Read the model definition and answer for the solid it produces. Units are mm, in the model's axes. Face numbers are marked on the shaded views. Coordinates: 2 decimals unless noted, no trailing zeros. Order: outer loops, then holes, each group sorted by start corner. A loop starts at its lowest first (then second) coordinate and runs counter-clockwise, first axis right, second up. Notation, with made-up numbers: (73, 71.5) -> (95, 71.5) arc R19 ccw to (95, 82.5) -> close; hole circle Ø9 at (-10.75, -17.75). An arc over 180 degrees is marked (long way). Answer as a JSON object with one key per item and string values. Group by question number.
1) Determine the mould class of the marked faces 1 and 2 for opening direction X: released by +X, released by -X, zero draft, split by the parting line, or undercut.
2) Section C-C on y = 119 is taken. Determine the outline of the cut face in (x, z), and give its area (3 significant figures).
3) Section A-A on x = 0 is taken. Determine the outline of the cut face in (y, z), and give its area (3 significant figures).
4) Given pin 1 (3 mm diameter, centred on y = 70.5, z = 4, fed in from -X); pin 2 (2 mm diameter, centred on x = 10, y = 101.5, fed in from +Z); pin 3 (1.5 mm diameter, centred on x = -7, y = 53, fed in from +Z), each flat-ended and moving along its own axis, determine where each tip first touches the part or whether it passes through.
5) Consider L1, parallel to X at y = 98, z = -0.25; L2, parallel to Z at x = 1.75, y = 81; L3, parallel to X at y = 50.5, z = 3.25. Determine where each line is inside the solid, lowest interval first.
6) Section B-B on z = 0 is taken. Determine the outline of the cut face in (x, y).
from build123d import *
from OCP.BRepFilletAPI import BRepFilletAPI_MakeChamfer

# Parameters (mm, degrees)
SKETCH1_R           = 15
BOSS_EXTRUDE1_DEPTH = 153.775561
SKETCH2_R           = 8.083843349
CUT_EXTRUDE1_DEPTH  = 156.231836815
CHAMFER1_SIZE       = 3.249874
CHAMFER1_SIZE2      = 2.3566


with BuildPart() as part:
    # Sketch1 → Boss-Extrude1 (new body)
    with BuildSketch(Plane(origin=(0, 0, 0), x_dir=(1, 0, 0), z_dir=(0, 1, 0))):
        with Locations(Location((0, 0, 0), (0, 0, 270))):
            Circle(SKETCH1_R)
    extrude(amount=BOSS_EXTRUDE1_DEPTH)

    # Sketch2 → Cut-Extrude1 (cut, through all)
    with BuildSketch(Plane(origin=(0, 0, 0), x_dir=(1, 0, 0), z_dir=(0, 1, 0))):
        with Locations(Location((0, 0, 0), (0, 0, 270))):
            Circle(SKETCH2_R)
    extrude(amount=CUT_EXTRUDE1_DEPTH, mode=Mode.SUBTRACT)

    # Chamfer1: one chamfer whose edges measure the first distance from different faces: ONE call of the kernel's chamfer builder (chamfer() names one face for all edges)
    chamfer1_edges_1 = [part.edges().sort_by_distance(p)[0] for p in [
        (0, 0, -15),
    ]]
    chamfer1_side_1 = [part.faces().sort_by_distance(p)[0] for p in [
        (0, 76.8877805, -15),
    ]]
    chamfer1_edges_2 = [part.edges().sort_by_distance(p)[0] for p in [
        (0, 153.775561, -15),
    ]]
    chamfer1_side_2 = [part.faces().sort_by_distance(p)[0] for p in [
        (0, 153.775561, -14.575735931),
    ]]
    chamfer1 = BRepFilletAPI_MakeChamfer(part.part.solid().wrapped)
    for e in chamfer1_edges_1:
        chamfer1.Add(CHAMFER1_SIZE, CHAMFER1_SIZE2, e.wrapped, chamfer1_side_1[0].wrapped)  # the first distance lies on this face
    for e in chamfer1_edges_2:
        chamfer1.Add(CHAMFER1_SIZE, CHAMFER1_SIZE2, e.wrapped, chamfer1_side_2[0].wrapped)  # the first distance lies on this face
    add(Compound.cast(chamfer1.Shape()), mode=Mode.REPLACE)


solid = part.part
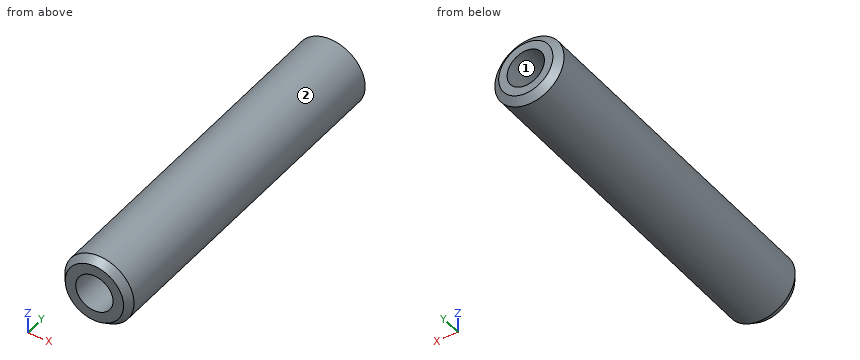
Worked answers:
{
 "1": {"face 1": "undercut", "face 2": "split by the parting line"},
 "2": {"outline": "circle Ø30 at (0, 0); hole circle Ø16.17 at (0, 0)", "area": "502 mm²"},
 "3": {"outline": "(0, -12.64) -> (3.25, -15) -> (151.42, -15) -> (153.78, -11.75) -> (153.78, -8.08) -> (0, -8.08) -> close; (0, 8.08) -> (153.78, 8.08) -> (153.78, 11.75) -> (151.42, 15) -> (3.25, 15) -> (0, 12.64) -> close", "area": "2,110 mm²"},
 "4": {"pin 1": "stops at x = -14.79", "pin 2": "stops at z = 12", "pin 3": "stops at z = 13.64"},
 "5": {"L1": "x = -15 to -8.08, 8.08 to 15", "L2": "z = -14.9 to -7.89, 7.89 to 14.9", "L3": "x = -14.64 to -7.4, 7.4 to 14.64"},
 "6": {"outline": "(-15, 3.25) -> (-12.64, 0) -> (-8.08, 0) -> (-8.08, 153.78) -> (-11.75, 153.78) -> (-15, 151.42) -> close; (8.08, 0) -> (12.64, 0) -> (15, 3.25) -> (15, 151.42) -> (11.75, 153.78) -> (8.08, 153.78) -> close"}
}
